Geometry check sheet. Reference: the model listing, model coordinates, mm. A direction names the side the tool comes from. Round coordinates to 2 decimals unless told otherwise and drop trailing zeros. Write each loop counter-clockwise with the first axis right and the second up, starting at its lowest first coordinate (ties: lowest second). Pieces come first, ordered by that corner, then holes.
Item 1: Cross-section at B-B (x = -0.75). Enter the section's corners in (y, z), then the cut area to 3 significant figures.
Item 2: Cross-section at A-A (z = 0). Enter the section's corners in (x, y) (3 decimals).
Item 3: Access from +Z, -Z, +X, -X, +Y, -Y to the whole of each face (thin tool, end or side, straight path). Record for faces 5 (the face through (-0.108, 2.806, 10.488)), 6 (the face through (2.003, 3.58, -0.631)).
Item 4: Scan lines: probe 1 along X at (y, z) = (2.55, 0) (3 decimals); probe 2 along Y at (x, z) = (1.65, -6.5); probe 3 along Z at (x, y) = (-0.1, 1.1). Record each from-to range of solid material in increasing order.
Item 5: Depth check by flat-ended pin: P1, Ø1.3, axis at x = -1, z = 1, coming from the -Y side; P2, Ø1, axis at x = 1, z = -4, coming from the +Y side; P3, Ø1.5, axis at y = 2.5, z = -6, coming from the +X side. Enter the tip coordinate at first touch or a pass-through.
Item 6: Cross-section at C-C (y = 1.8). Enter the section's corners in (x, z) (3 decimals), then the cut area to 3 significant figures.
Item 7: Draft check along Z on faces 1 (the face through (-0.108, 2.806, 8.488)), 2 (the face through (-2.932, 1.489, -0.129)), 3 (the face through (-2.244, 2.806, -6.335)), 4 (the face through (2.003, 1.159, 0.631)). Enter one of: pulls with the +Z half, pulls with the -Z half, needs draft (parallel to the pull), parting line crosses it, or undercut.
Item 8: Cross-section at D-D (z = -8). Enter the section's corners in (x, y).
from build123d import *

# Parameters (mm, degrees)
SKETCH1_R           = 2.935
BOSS_EXTRUDE2_DEPTH = 3.25
SKETCH2_R           = 0.5
BOSS_EXTRUDE3_DEPTH = 0.9
SKETCH3_R           = 2.935
BOSS_EXTRUDE4_DEPTH = 0.65
SKETCH4_R           = 2.1
CUT_EXTRUDE1_DEPTH  = 0.65
SKETCH5_R           = 1
CUT_EXTRUDE2_DEPTH  = 5.65
SKETCH6_R           = 2.1
CUT_EXTRUDE3_DEPTH  = 2.35


with BuildPart() as part:
    # Sketch1 → Boss-Extrude2 (new body)
    with BuildSketch(Plane(origin=(0, 0, 0), x_dir=(1, 0, 0), z_dir=(0, 1, 0))):
        Circle(SKETCH1_R)
    extrude(amount=BOSS_EXTRUDE2_DEPTH)

    # Sketch2 → Boss-Extrude3 (add)
    with BuildSketch(Plane(origin=(0, 3.25, 0), x_dir=(1, 0, 0), z_dir=(0, 1, 0))):
        with BuildLine():
            ThreePointArc((-2.916780846, 0.32651875), (-1.956513796, 2.18775656), (0, 2.935))
            ThreePointArc((0, 2.935), (1.956513796, 2.18775656), (2.916780846, 0.32651875))
            Line((2.916780846, 0.32651875), (1.590067923, 12.178))
            ThreePointArc((1.590067923, 12.178), (0, 13.6), (-1.590067923, 12.178))
            Line((-1.590067923, 12.178), (-2.916780846, 0.32651875))
        make_face()
        with BuildLine():
            ThreePointArc((0, 8.5), (0.5, 8), (0, 7.5))
            ThreePointArc((0, 7.5), (-0.5, 8), (0, 8.5))
        make_face(mode=Mode.SUBTRACT)
        with Locations((0, 10)):
            Circle(SKETCH2_R, mode=Mode.SUBTRACT)
        with Locations((0, 12)):
            Circle(SKETCH2_R, mode=Mode.SUBTRACT)
        with BuildLine():
            Line((1.590067923, -12.178), (2.916780846, -0.32651875))
            ThreePointArc((2.916780846, -0.32651875), (0, -2.935), (-2.916780846, -0.32651875))
            Line((-2.916780846, -0.32651875), (-1.590067923, -12.178))
            ThreePointArc((-1.590067923, -12.178), (0, -13.6), (1.590067923, -12.178))
        make_face()
        with Locations((0, -12)):
            Circle(SKETCH2_R, mode=Mode.SUBTRACT)
        with Locations((0, -10)):
            Circle(SKETCH2_R, mode=Mode.SUBTRACT)
        with Locations((0, -8)):
            Circle(SKETCH2_R, mode=Mode.SUBTRACT)
    extrude(amount=-BOSS_EXTRUDE3_DEPTH)

    # Sketch3 → Boss-Extrude4 (add)
    with BuildSketch(Plane(origin=(0, 3.25, 0), x_dir=(1, 0, 0), z_dir=(0, 1, 0))):
        Circle(SKETCH3_R)
    extrude(amount=BOSS_EXTRUDE4_DEPTH)

    # Sketch4 → Cut-Extrude1 (cut)
    with BuildSketch(Plane(origin=(0, 3.9, 0), x_dir=(1, 0, 0), z_dir=(0, 1, 0))):
        Circle(SKETCH4_R)
    extrude(amount=-CUT_EXTRUDE1_DEPTH, mode=Mode.SUBTRACT)

    # Sketch5 → Cut-Extrude2 (cut)
    with BuildSketch(Plane(origin=(0, 3.25, 0), x_dir=(1, 0, 0), z_dir=(0, 1, 0))):
        Circle(SKETCH5_R)
    extrude(amount=-CUT_EXTRUDE2_DEPTH, mode=Mode.SUBTRACT)

    # Sketch6 → Cut-Extrude3 (cut)
    with BuildSketch(Plane.XZ):
        Circle(SKETCH6_R)
    extrude(amount=-CUT_EXTRUDE3_DEPTH, mode=Mode.SUBTRACT)


solid = part.part
Resolved:
1. outline: (0, -2.84) - (2.35, -2.84) - (2.35, -13.41) - (3.25, -13.41) - (3.25, -2.84) - (3.9, -2.84) - (3.9, -1.96) - (3.25, -1.96) - (3.25, -0.66) - (2.35, -0.66) - (2.35, -1.96) - (0, -1.96) - close; (0, 1.96) - (2.35, 1.96) - (2.35, 0.66) - (3.25, 0.66) - (3.25, 1.96) - (3.9, 1.96) - (3.9, 2.84) - (3.25, 2.84) - (3.25, 13.41) - (2.35, 13.41) - (2.35, 2.84) - (0, 2.84) - close
1. area: 28.2 mm2
2. outline: (-2.935, 0) - (-2.1, 0) - (-2.1, 2.35) - (-1, 2.35) - (-1, 3.25) - (-2.1, 3.25) - (-2.1, 3.9) - (-2.935, 3.9) - close; (1, 2.35) - (2.1, 2.35) - (2.1, 0) - (2.935, 0) - (2.935, 3.9) - (2.1, 3.9) - (2.1, 3.25) - (1, 3.25) - close
3. face 5: +Y, -Y
3. face 6: +Y
4. probe 1: x = -2.935 to -1, 1 to 2.935
4. probe 2: y = 2.35 to 3.25
4. probe 3: z = -2.93 to -2.1, 2.1 to 2.93
5. P1: stops at y = 2.35
5. P2: stops at y = 3.25
5. P3: stops at x = 2.37
6. outline: circle Ø5.87 at (0, 0); hole circle Ø4.2 at (0, 0)
6. area: 13.2 mm2
7. face 1: undercut
7. face 2: parting line crosses it
7. face 3: pulls with the -Z half
7. face 4: undercut
8. outline: (-2.06, 2.35) - (-0.5, 2.35) - (-0.5, 3.25) - (-2.06, 3.25) - close; (0.5, 2.35) - (2.06, 2.35) - (2.06, 3.25) - (0.5, 3.25) - close
